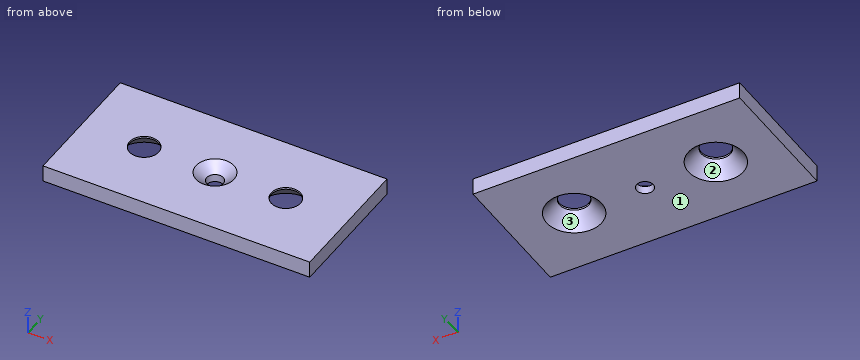
from build123d import *

# Parameters (mm, degrees)
SKETCH1_W                                         = 50.8
SKETCH1_H                                         = 25.4
BOSS_EXTRUDE1_DEPTH                               = 3.175
CSK_FOR_6_FLAT_HEAD_MACHINE_SCREW_100_D           = 3.175
CSK_FOR_6_FLAT_HEAD_MACHINE_SCREW_100_DEPTH       = 25.4
CSK_FOR_6_FLAT_HEAD_MACHINE_SCREW_100_CSINK_D     = 7.239
CSK_FOR_6_FLAT_HEAD_MACHINE_SCREW_100_CSINK_ANGLE = 100
CSK_FOR_6_FLAT_HEAD_MACHINE_SCREW_100_TIP         = 0.953866233


# Read off the part's stored shape, not the designer's step: CSK for #6 Flat Head Machine Screw (100)2
with BuildPart() as part:
    # Sketch1 → Boss-Extrude1 (new body)
    with BuildSketch(Plane.XY):
        with Locations((25.4, 12.7)):
            Rectangle(SKETCH1_W, SKETCH1_H)
    extrude(amount=BOSS_EXTRUDE1_DEPTH)

    # CSK for _6 Flat Head Machine Screw _100
    with Locations(Plane.XY.offset(3.175)):
        with Locations((25.4, 12.7)):
            CounterSinkHole(CSK_FOR_6_FLAT_HEAD_MACHINE_SCREW_100_D / 2, CSK_FOR_6_FLAT_HEAD_MACHINE_SCREW_100_CSINK_D / 2, depth=CSK_FOR_6_FLAT_HEAD_MACHINE_SCREW_100_DEPTH, counter_sink_angle=CSK_FOR_6_FLAT_HEAD_MACHINE_SCREW_100_CSINK_ANGLE)
            with Locations((0, 0, -(CSK_FOR_6_FLAT_HEAD_MACHINE_SCREW_100_DEPTH + CSK_FOR_6_FLAT_HEAD_MACHINE_SCREW_100_TIP / 2))):  # 118° drill point
                Cone(0, CSK_FOR_6_FLAT_HEAD_MACHINE_SCREW_100_D / 2, CSK_FOR_6_FLAT_HEAD_MACHINE_SCREW_100_TIP, mode=Mode.SUBTRACT)

    # CSK for _6 Flat Head Machine Screw _ 2 o → CSK for _6 Flat Head Machine Screw _ 2 (revolve, cut)
    with BuildSketch(Plane(origin=(11.90625, 12.7, 0), x_dir=(1, 0, 0), z_dir=(0, -1, 0))):
        Polygon((2.778125, 2.823320423), (2.778125, 3.175), (0, 3.175), (0, 0), (5.2324, 0), align=None)
    revolve(axis=Axis((11.90625, 12.7, 0), (0, 0, 1)), mode=Mode.SUBTRACT)

    # CSK for _6 Flat Head Machine Screw _ 3 → CSK for _6 Flat Head Machine Screw _ 2 2 (revolve, cut)
    with BuildSketch(Plane(origin=(38.89375, 12.7, 0), x_dir=(1, 0, 0), z_dir=(0, -1, 0))):
        Polygon((2.778125, 2.823320423), (2.778125, 3.175), (0, 3.175), (0, 0), (5.2324, 0), align=None)
    revolve(axis=Axis((38.89375, 12.7, 0), (0, 0, 1)), mode=Mode.SUBTRACT)


solid = part.part
Can you work these out from the model? Positions are in its coordinate system, mm. Face numbers are marked on the shaded views. Round coordinates to 2 decimals unless told otherwise and drop trailing zeros. Order: outer loops, then holes, each group sorted by start corner. A loop starts at its lowest first (then second) coordinate and runs counter-clockwise, first axis right, second up. Notation, with made-up numbers: (23.25, 23.25) - (47.25, 23.25) arc R29 ccw to (47.25, 57.25) - close; hole circle Ø7 at (-18.5, 66). An arc over 180 degrees is marked (long way). Answer in a Markdown table with one row per item.
(1) Suppose I cut it at B-B, the plane x = 25.4. Please give me the cut outline in (y, z) (1 decimal).
From the geometry:
| item | result |
|---|---|
| outline | (0, 0) - (11.1, 0) - (11.1, 1.5) - (9.1, 3.2) - (0, 3.2) - close; (14.3, 0) - (25.4, 0) - (25.4, 3.2) - (16.3, 3.2) - (14.3, 1.5) - close |
(2) Suppose I cut it at C-C, the plane z = 0.75. Please give me the cut outline in (x, y) (1 decimal), plus the area to 3 significant figures.
From the geometry:
| item | result |
|---|---|
| outline | (0, 0) - (50.8, 0) - (50.8, 25.4) - (0, 25.4) - close; hole circle Ø9.2 at (11.9, 12.7); hole circle Ø3.2 at (25.4, 12.7); hole circle Ø9.2 at (38.9, 12.7) |
| area | 1,150 mm2 |
(3) Suppose I cut it at A-A, the plane y = 12.7. Count the separate pieces of the cut face and the enclosed holes in it, plus the area to 3 significant figures.
From the geometry:
| item | result |
|---|---|
| separate pieces | 4 |
| enclosed holes | 0 |
| area | 98.6 mm2 |
(4) If we mould it in two halves opening along X, with no side actions, what happens to the marked faces 1, 2 and 3? For each: released by +X, released by -X, zero draft, split by the parting line, or undercut.
From the geometry:
| item | result |
|---|---|
| face 1 | zero draft |
| face 2 | undercut |
| face 3 | undercut |
(5) For P1, Ø4.5, axis at x = 11.91, y = 12.7, coming from the -Z side, with a flat end and sliding along its axis, tell me the tip position at first contact or that it passes through.
From the geometry:
| item | result |
|---|---|
| P1 | passes through |
(6) Please list where these lines run through material, in increasing order: L1, parallel to Y at x = 25.4, z = 0.85; L2, parallel to X at y = 10.75, z = 2.3; L3, parallel to X at y = 11.25, z = 0.9. Write a range as from..to.
From the geometry:
| item | result |
|---|---|
| L1 | y = 0..11.11, 14.29..25.4 |
| L2 | x = 0..9.33, 14.49..23.72, 27.08..36.31, 41.47..50.8 |
| L3 | x = 0..7.7, 16.11..24.75, 26.05..34.69, 43.1..50.8 |
